Geometry check sheet. Reference: drawing and pictorial views, mm from the part's lowest x, y, z. A direction names the side the tool comes from. Give positions to 0.01 mm unless a question says otherwise; leave off trailing zeros. Loops run counter-clockwise (first coordinate to the right, second up) from the corner with the lowest first, then second, coordinate; pieces in that order, holes last. Notation, with made-up numbers: M 11,75.5 L 33,75.5 A19 cw 33,92.5 Z; hole C -7.5,73 d10. An arc over 180 degrees is marked long. Use CSV: the item, a comma, the result in double quotes.
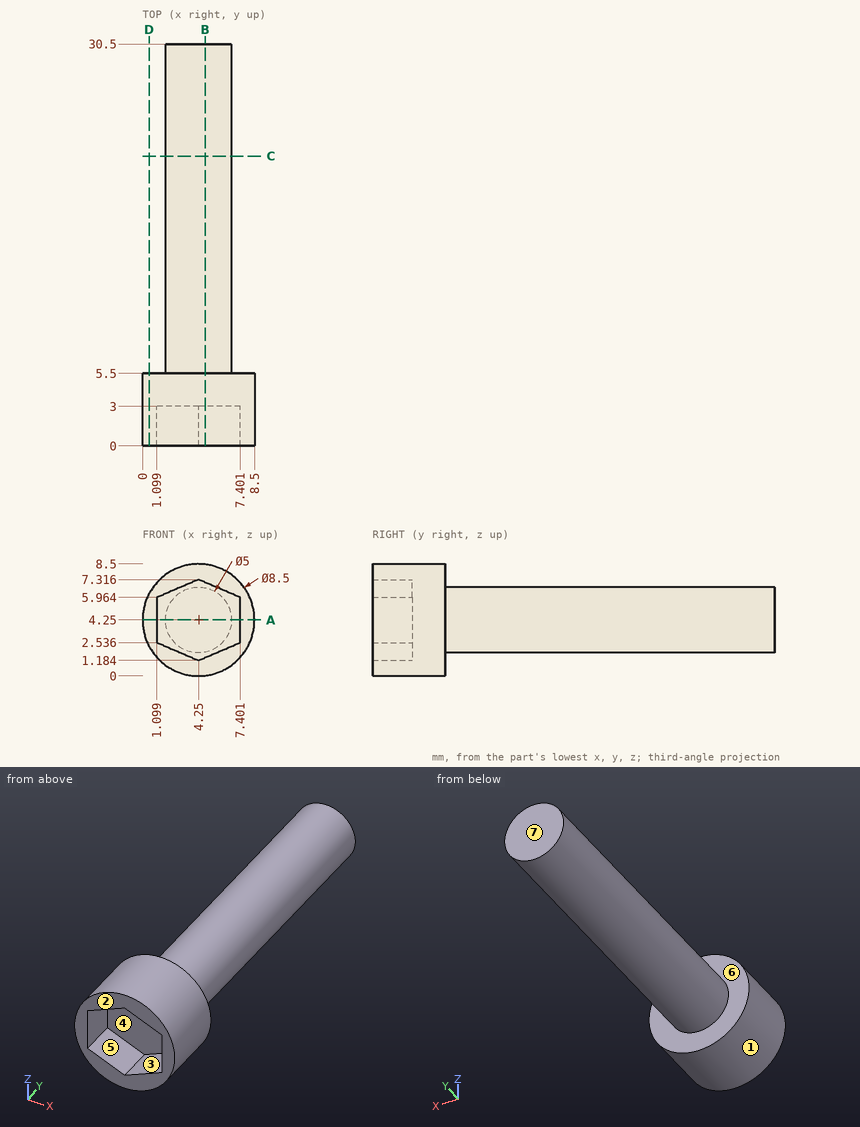
(1) Section check B-B on x = 4.75. Record the cut outline in (y, z), plus the area to 3 significant figures.
Calculated:
outline,"M 0,0.03 L 5.5,0.03 L 5.5,1.8 L 30.5,1.8 L 30.5,6.7 L 5.5,6.7 L 5.5,8.47 L 0,8.47 L 0,7.1 L 3,7.1 L 3,1.4 L 0,1.4 Z"
area,"152 mm²"
(2) Mould release check, pull along X, two halves, no side actions. Record for the marked faces 1, 2, 3 and 4: released by +X, released by -X, zero draft, split by the parting line, or undercut.
Calculated:
face 1,"split by the parting line"
face 2,"zero draft"
face 3,"undercut"
face 4,"undercut"
(3) Section check D-D on x = 0.5. Record the cut outline in (y, z).
Calculated:
outline,"M 0,2.25 L 5.5,2.25 L 5.5,6.25 L 0,6.25 Z"
(4) Scan lines: L1, parallel to Y at x = 5.75, z = 0.75; L2, parallel to Z at x = 1.5, y = 1.5 (1 decimal); L3, parallel to Y at x = 4.25, z = 5.5. Record each from-to range of solid material in increasing order. Write a range as from..to.
Calculated:
L1,"y = 0..5.5"
L2,"z = 1..2.4, 6.1..7.5"
L3,"y = 3..30.5"
(5) Section check A-A on z = 4.25. Record the cut outline in (x, y), plus the area to 3 significant figures.
Calculated:
outline,"M 0,0 L 1.1,0 L 1.1,3 L 7.4,3 L 7.4,0 L 8.5,0 L 8.5,5.5 L 6.75,5.5 L 6.75,30.5 L 1.75,30.5 L 1.75,5.5 L 0,5.5 Z"
area,"153 mm²"
(6) Depth check by flat-ended pin: pin 1 Ø3 at (x, y) = (6, 4.5) entering from +Z; pin 2 Ø1.5 at (y, z) = (27, 5) entering from +X; pin 3 Ø5 at (y, z) = (25.5, 3) entering from -X. Enter the tip coordinate at first touch or a pass-through.
Calculated:
pin 1,"stops at z = 8.49"
pin 2,"stops at x = 6.75"
pin 3,"stops at x = 1.75"
(7) Section check C-C on y = 22. Record the cut outline in (x, z), plus the area to 3 significant figures.
Calculated:
outline,"C 4.25,4.25 d5"
area,"19.6 mm²"
(8) Tool access check on the marked faces 5, 6 and 7. Record the directions out of +Z, -Z, +X, -X, +Y, -Y that give a thin tool (end or side, any length) a straight path to the whole face; none if there is none.
Calculated:
face 5,"-Y"
face 6,"+Y"
face 7,"+Z, -Z, +X, -X, +Y"
